from build123d import *

# Parameters (mm, degrees)
SKETCH_2_W          = 60
SKETCH_2_H          = 15
SKETCH_2_R          = 1.3
EXTRUDE_1_DEPTH     = 10
SKETCH_3_W          = 25
SKETCH_3_H          = 15
EXTRUDE_2_DEPTH     = 70
EXTRUDE_3_DEPTH     = 2
SKETCH_6_W          = 10
SKETCH_6_H          = 5
EXTRUDE_4_DEPTH     = 15
SKETCH_7_R          = 2
CUT_EXTRUDE_1_DEPTH = 81.970673704


with BuildPart() as part:
    # 草圖2 → 填料-伸長1 (new body)
    with BuildSketch(Plane(origin=(0, 0, 0), x_dir=(1, 0, 0), z_dir=(0, 1, 0))):
        Rectangle(SKETCH_2_W, SKETCH_2_H)
        with Locations(Location((-22.5, 0, 0), (0, 0, 270))):
            Circle(SKETCH_2_R, mode=Mode.SUBTRACT)
        with Locations(Location((22.5, 0, 0), (0, 0, 90))):
            Circle(SKETCH_2_R, mode=Mode.SUBTRACT)
    extrude(amount=EXTRUDE_1_DEPTH)

    # 草圖3 → 填料-伸長2 (add)
    with BuildSketch(Plane(origin=(0, 10, 0), x_dir=(1, 0, 0), z_dir=(0, 1, 0))):
        Rectangle(SKETCH_3_W, SKETCH_3_H)
    extrude(amount=EXTRUDE_2_DEPTH)

    # 草圖5 → 填料-伸長3 (add)
    with BuildSketch(Plane(origin=(0, 0, -7.5), x_dir=(-1, 0, 0), z_dir=(0, 0, -1))):
        Polygon((-30, 10), (-12.5, 27.5), (-12.5, 10), align=None)
        Polygon((12.5, 27.5), (12.5, 10), (30, 10), align=None)
    extrude(amount=-EXTRUDE_3_DEPTH)

    # 草圖6 → 填料-伸長4 (add)
    with BuildSketch(Plane.XY.offset(7.5)):
        with Locations((-35, 7.5)):
            Rectangle(SKETCH_6_W, SKETCH_6_H)
    extrude(amount=-EXTRUDE_4_DEPTH)

    # 草圖7 → 除料-伸長1 (cut, through all)
    with BuildSketch(Plane(origin=(0, 10, 0), x_dir=(1, 0, 0), z_dir=(0, 1, 0))):
        with Locations(Location((-35, 0, 0), (0, 0, 270))):
            Circle(SKETCH_7_R)
    extrude(amount=-CUT_EXTRUDE_1_DEPTH, mode=Mode.SUBTRACT)


solid = part.part
Verification items for the finished model (mm, model axes). A direction names the side the tool comes from. Coordinates: 2 decimals unless noted, no trailing zeros. Order: outer loops, then holes, each group sorted by start corner. A loop starts at its lowest first (then second) coordinate and runs counter-clockwise, first axis right, second up. Notation, with made-up numbers: (32.5, 89) -> (71.5, 89) arc R12 ccw to (71.5, 98) -> close; hole circle Ø5 at (-14, 67). An arc over 180 degrees is marked (long way). Use CSV: the item, a comma, the result in double quotes. Start each with the question number.
Q1. Section check A-A, the plane x = -35. Record the cut outline in (y, z), and give its area (3 significant figures).
Q2. Section check D-D, the plane x = -22.5. Record the cut outline in (y, z), and give its area (3 significant figures).
Q3. Draft check along Z on faces 1 (the flat face through (-26, 10, 0)), 2 (the flat face through (17, 15, -5.5)), 3 (the cylindrical face through (23.77, 4.93, 0.28)), 4 (the cylindrical face through (-23.77, 4.93, -0.28)). Enter one of: +Z half, -Z half, draft (parallel to the pull), parting line (faces both ways), or undercut.
Q4. Depth check by flat-ended pin: P1, Ø3.5, axis at x = -22.5, z = 0, coming from the +Y side; P2, Ø5.5, axis at x = 20.5, y = 16, coming from the +Z side; P3, Ø4, axis at y = 13, z = -5, coming from the -X side; P4, Ø2.5, axis at x = -35, z = 0, coming from the -Y side. Enter the tip coordinate at first touch or a pass-through.
Q5. Tool access check on faces 5 (the flat face through (-30, 2, 0)), 6 (the flat face through (-17, 15, -5.5)), 7 (the flat face through (12.5, 45, 0)). Record the directions out of +Z, -Z, +X, -X, +Y, -Y that give a thin tool (end or side, any length) a straight path to the whole face; none if there is none.
Q6. Section check C-C, the plane y = 14. Record the cut outline in (x, z).
Q7. Section check B-B, the plane z = 0. Record the cut outline in (x, y).
Q8. Thickness scan on line 1 along X through (y, z) = (8, 0); line 2 along X through (y, z) = (2.75, 0); line 3 along Y through (x, z) = (-23.5, -5.25). Record the ranges inside material, lowest first.
Returned:
1,outline,"(5, -7.5) -> (10, -7.5) -> (10, -2) -> (5, -2) -> close; (5, 2) -> (10, 2) -> (10, 7.5) -> (5, 7.5) -> close"
1,area,"55.0 mm^2"
2,outline,"(0, -7.5) -> (17.5, -7.5) -> (17.5, -5.5) -> (10, -5.5) -> (10, -1.3) -> (0, -1.3) -> close; (0, 1.3) -> (10, 1.3) -> (10, 7.5) -> (0, 7.5) -> close"
2,area,"139 mm^2"
3,face 1,"draft"
3,face 2,"+Z half"
3,face 3,"undercut"
3,face 4,"undercut"
4,P1,"stops at y = 10"
4,P2,"stops at z = -5.5"
4,P3,"stops at x = -28.94"
4,P4,"passes through"
5,face 5,"+Z, -Z, -X, -Y"
5,face 6,"+Z, -X, +Y"
5,face 7,"+Z, +X, +Y"
6,outline,"(-26, -7.5) -> (26, -7.5) -> (26, -5.5) -> (12.5, -5.5) -> (12.5, 7.5) -> (-12.5, 7.5) -> (-12.5, -5.5) -> (-26, -5.5) -> close"
7,outline,"(-40, 5) -> (-37, 5) -> (-37, 10) -> (-40, 10) -> close; (-33, 5) -> (-30, 5) -> (-30, 0) -> (-23.8, 0) -> (-23.8, 10) -> (-33, 10) -> close; (-21.2, 0) -> (21.2, 0) -> (21.2, 10) -> (12.5, 10) -> (12.5, 80) -> (-12.5, 80) -> (-12.5, 10) -> (-21.2, 10) -> close; (23.8, 0) -> (30, 0) -> (30, 10) -> (23.8, 10) -> close"
8,line 1,"x = -40 to -37, -33 to -23.8, -21.2 to 21.2, 23.8 to 30"
8,line 2,"x = -30 to -23.8, -21.2 to 21.2, 23.8 to 30"
8,line 3,"y = 0 to 10"
